The listing builds one solid part. Answer for the finished solid, in the listing's coordinates (mm). A direction names the side the tool comes from. Round coordinates to 2 decimals unless told otherwise and drop trailing zeros. Write each loop counter-clockwise with the first axis right and the second up, starting at its lowest first coordinate (ties: lowest second). Pieces come first, ordered by that corner, then holes.
from build123d import *

# Parameters (mm, degrees)
PAD_DEPTH       = 5
POCKET_DEPTH    = 4
POCKET004_DEPTH = 5
FILLET_R        = 1
FILLET001_R     = 1
FILLET002_R     = 0.3
FILLET003_R     = 0.3
SKETCH012_W     = 12.408569
SKETCH012_H     = 1.7372
POCKET007_DEPTH = 2


with BuildPart() as part:
    # Sketch → Pad (new body)
    with BuildSketch(Plane.XY):
        with BuildLine():
            Line((-10.302154, -6.75), (-10.302154, 6.75))
            Line((-10.302154, 6.75), (4.697846, 6.75))
            ThreePointArc((4.697846, -6.75), (21.401934, 0), (4.697846, 6.75))
            Line((-10.302154, -6.75), (4.697846, -6.75))
        make_face()
    extrude(amount=PAD_DEPTH)

    # Sketch001 (on Face6 of Pad) → Pocket (cut)
    with BuildSketch(Plane.XY.offset(5)):
        with BuildLine():
            Line((-9.568426, -6.285917), (4.972526, -6.285917))
            ThreePointArc((4.972526, -6.285917), (20.334041, -0.01843), (4.970857, 6.244966))
            Line((-9.568426, 6.244966), (4.970857, 6.244966))
            Line((-9.568426, -6.285917), (-9.568426, 6.244966))
        make_face()
    extrude(amount=-POCKET_DEPTH, mode=Mode.SUBTRACT)

    # Sketch010 (on Face11 of Pocket) → Pocket004 (cut)
    with BuildSketch(Plane.XY.offset(1)):
        with BuildLine():
            ThreePointArc((16.954988, 6.278391), (13.004004, 8.225263), (8.611476, 7.899254))
            Line((8.611476, 7.899254), (9.109037, 6.707427))
            ThreePointArc((16.036381, 5.369056), (12.751013, 6.961134), (9.109037, 6.707427))
            Line((16.954988, 6.278391), (16.036381, 5.369056))
        make_face()
        with BuildLine():
            ThreePointArc((8.677646, -7.709712), (12.991395, -8.023159), (16.861761, -6.092627))
            Line((15.900234, -5.234123), (16.861761, -6.092627))
            ThreePointArc((9.154517, -6.521003), (12.69888, -6.776571), (15.900234, -5.234123))
            Line((8.677646, -7.709712), (9.154517, -6.521003))
        make_face()
    extrude(amount=-POCKET004_DEPTH, mode=Mode.SUBTRACT)

    # Fillet
    fillet_edges = [part.edges().sort_by_distance(p)[0] for p in [
        (-2.802154, -6.75, 0),
    ]]
    fillet(fillet_edges, radius=FILLET_R)

    # Fillet001
    fillet001_edges = [part.edges().sort_by_distance(p)[0] for p in [
        (-2.802154, 6.75, 0),
    ]]
    fillet(fillet001_edges, radius=FILLET001_R)

    # Fillet002
    fillet002_edges = [part.edges().sort_by_distance(p)[0] for p in [
        (12.751013, 6.961134, 0),
    ]]
    fillet(fillet002_edges, radius=FILLET002_R)

    # Fillet003
    fillet003_edges = [part.edges().sort_by_distance(p)[0] for p in [
        (12.69888, -6.776571, 0),
    ]]
    fillet(fillet003_edges, radius=FILLET003_R)

    # Sketch012 (on Face10 of Fillet003) → Pocket007 (cut)
    with BuildSketch(Plane(origin=(-10.302154, 0, 0), x_dir=(0, -1, 0), z_dir=(-1, 0, 0))):
        with Locations((0.011792, 2.757287)):
            Rectangle(SKETCH012_W, SKETCH012_H)
    extrude(amount=-POCKET007_DEPTH, mode=Mode.SUBTRACT)


solid = part.part
1. Straight lines are drawn through the part: line 1 along Y through (x, z) = (2, 2); line 2 along Z through (x, y) = (4, -1.75); line 3 along X through (y, z) = (-5.5, 1.35). For each, find the intervals that lie inside material, in ascending order.
Geometry says:
line 1: y = -6.75 to -6.29, 6.24 to 6.75
line 2: z = 0 to 1
line 3: x = -10.3 to -9.57, 18.46 to 19.7
2. Section C-C on z = 2.25 is taken. Determine the outline of the cut face in (x, y), plus the area to 3 significant figures.
Geometry says:
outline: (-10.3, -6.75) - (4.7, -6.75) arc R9.72 ccw (long way) to (4.7, 6.75) - (-10.3, 6.75) - (-10.3, 6.19) - (-9.57, 6.19) - (-9.57, 6.24) - (4.97, 6.24) arc R8.96 cw (long way) to (4.97, -6.29) - (-9.57, -6.29) - (-9.57, -6.22) - (-10.3, -6.22) - close
area: 52.3 mm2
3. A tool of negligible diameter and unlimited length cuts with its end or side. For faces 5 (the face through (-2.697, -6.465, 0.301)), 6 (the face through (12.8, 6.95, 0.65)), 7 (the face through (-2, -6.286, 3)), 8 (the face through (4.4, 6.5, 5)), 9 (the face through (6, 0, 0)), from which of +Z, -Z, +X, -X, +Y, -Y can it reach the whole face along a straight path? Write none if from no direction.
Geometry says:
face 5: -Z, -X, -Y
face 6: +Z, -Z
face 7: +Z
face 8: +Z, +X, -X, +Y, -Y
face 9: -Z, +X, -X, +Y, -Y
4. Section B-B on y = 0 is taken. Determine the outline of the cut face in (x, z).
Geometry says:
outline: (-10.3, 0) - (21.4, 0) - (21.4, 5) - (20.33, 5) - (20.33, 1) - (-9.57, 1) - (-9.57, 1.89) - (-10.3, 1.89) - close; (-10.3, 3.63) - (-9.57, 3.63) - (-9.57, 5) - (-10.3, 5) - close
5. Section A-A on z = 4.55 is taken. Determine the outline of the cut face in (x, y), plus the area to 3 significant figures.
Geometry says:
outline: (-10.3, -6.75) - (4.7, -6.75) arc R9.72 ccw (long way) to (4.7, 6.75) - (-10.3, 6.75) - close; hole (-9.57, -6.29) - (4.97, -6.29) arc R8.96 ccw (long way) to (4.97, 6.24) - (-9.57, 6.24) - close
area: 61.4 mm2
6. Section D-D on x = 18 is taken. Determine the outline of the cut face in (y, z), plus the area to 3 significant figures.
Geometry says:
outline: (-7.38, 0) - (7.38, 0) - (7.38, 5) - (6.01, 5) - (6.01, 1) - (-6.05, 1) - (-6.05, 5) - (-7.38, 5) - close
area: 25.6 mm2
7. Given pin 1 (5.5 mm diameter, centred on x = 8.5, y = -4, fed in from +Z); pin 2 (1.5 mm diameter, centred on x = 1, z = 1.5, fed in from -Y); pin 3 (1.5 mm diameter, centred on x = 0.5, z = 4, fed in from +Y), each flat-ended and moving along its own axis, determine where each tip first touches the part or whether it passes through.
Geometry says:
pin 1: stops at z = 1
pin 2: stops at y = -6.75
pin 3: stops at y = 6.75
8. For a pull along Y with two mould halves and no side action, classify faces 1 (the face through (5, 0, 1)), 2 (the face through (-3, 6.75, 3)), 3 (the face through (-3, -6.75, 3)), 4 (the face through (-2, 6.245, 3)) as released by +Y, released by -Y, zero draft, split by the parting line, or undercut.
Geometry says:
face 1: undercut
face 2: released by +Y
face 3: released by -Y
face 4: undercut
